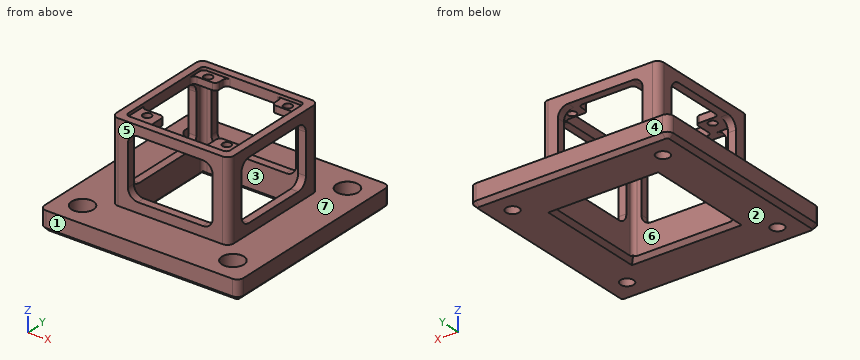
from build123d import *

# Parameters (mm, degrees)
SKETCH2_W                                    = 100
SKETCH2_H                                    = 100
SKETCH2_W_2                                  = 51.2
SKETCH2_H_2                                  = 51.2
BOSS_EXTRUDE1_DEPTH                          = 10
CBORE_FOR_M6_HEX_SOCKET_HEAD_CAP_SCR_2_COUNT = 2
CBORE_FOR_M6_HEX_SOCKET_HEAD_CAP_SCR_2_PITCH = 75.6
CBORE_FOR_M6_HEX_SOCKET_HEAD_CAP_SCR_3_COUNT = 2
CBORE_FOR_M6_HEX_SOCKET_HEAD_CAP_SCR_3_PITCH = 106.914545315
CBORE_FOR_M6_HEX_SOCKET_HEAD_CAP_SCR_4_COUNT = 2
CBORE_FOR_M6_HEX_SOCKET_HEAD_CAP_SCR_4_PITCH = 75.6
SKETCH7_W                                    = 59
SKETCH7_H                                    = 59
SKETCH7_W_2                                  = 51.2
SKETCH7_H_2                                  = 51.2
BOSS_EXTRUDE2_DEPTH                          = 40
SKETCH8_W                                    = 11.608814293
SKETCH8_H                                    = 6.4
SKETCH8_R                                    = 2.1
BOSS_EXTRUDE3_DEPTH                          = 5
FILLET1_R                                    = 3.2
SKETCH11_W                                   = 42.6
SKETCH11_H                                   = 30
CUT_EXTRUDE2_DEPTH                           = 107.396663482
SKETCH12_W                                   = 42.6
SKETCH12_H                                   = 30
CUT_EXTRUDE3_DEPTH                           = 107.396663482
FILLET3_R                                    = 5
FILLET4_R                                    = 5
CHAMFER2_SIZE                                = 2
CHAMFER3_SIZE                                = 2
SKETCH13_W                                   = 51.2
SKETCH13_H                                   = 51.2
CUT_EXTRUDE4_DEPTH                           = 1.5
FILLET5_R                                    = 2


with BuildPart() as part:
    # Sketch2 → Boss-Extrude1 (new body)
    with BuildSketch(Plane(origin=(0, 0, 0), x_dir=(0, 1, 0), z_dir=(0, 0, 1))):
        Rectangle(SKETCH2_W, SKETCH2_H)
        Rectangle(SKETCH2_W_2, SKETCH2_H_2, mode=Mode.SUBTRACT)
    extrude(amount=BOSS_EXTRUDE1_DEPTH)

    # Sketch6 → CBORE for M6 Hex Socket Head Cap Screw1 (revolve, cut)
    with BuildSketch(Plane(origin=(-37.8, 37.8, 10), x_dir=(0, -1, 0), z_dir=(1, 0, 0))):
        Polygon((0, 0), (0, 10), (3.3, 10), (3.3, 6.4), (5.5, 6.4), (5.5, 0.025), (5.525, 0), align=None)
    cbore_for_m6_hex_socket_head_cap_screw1 = revolve(axis=Axis((-37.8, 37.8, 16.35), (0, 0, -1)), mode=Mode.SUBTRACT)

    # CBORE for M6 Hex Socket Head Cap Scr 2: CBORE for M6 Hex Socket Head Cap Screw1 ×2
    with Locations(*[(i * CBORE_FOR_M6_HEX_SOCKET_HEAD_CAP_SCR_2_PITCH, 0, 0) for i in range(1, CBORE_FOR_M6_HEX_SOCKET_HEAD_CAP_SCR_2_COUNT)]):
        add(cbore_for_m6_hex_socket_head_cap_screw1, mode=Mode.SUBTRACT)

    # CBORE for M6 Hex Socket Head Cap Scr 3: CBORE for M6 Hex Socket Head Cap Screw1 ×2
    with Locations(*[Vector(0.7071067811865475, -0.7071067811865476, 0) * (i * CBORE_FOR_M6_HEX_SOCKET_HEAD_CAP_SCR_3_PITCH) for i in range(1, CBORE_FOR_M6_HEX_SOCKET_HEAD_CAP_SCR_3_COUNT)]):
        add(cbore_for_m6_hex_socket_head_cap_screw1, mode=Mode.SUBTRACT)

    # CBORE for M6 Hex Socket Head Cap Scr 4: CBORE for M6 Hex Socket Head Cap Screw1 ×2
    with Locations(*[(0, -i * CBORE_FOR_M6_HEX_SOCKET_HEAD_CAP_SCR_4_PITCH, 0) for i in range(1, CBORE_FOR_M6_HEX_SOCKET_HEAD_CAP_SCR_4_COUNT)]):
        add(cbore_for_m6_hex_socket_head_cap_screw1, mode=Mode.SUBTRACT)

    # Sketch7 → Boss-Extrude2 (add)
    with BuildSketch(Plane.XY.offset(10)):
        Rectangle(SKETCH7_W, SKETCH7_H)
        Rectangle(SKETCH7_W_2, SKETCH7_H_2, mode=Mode.SUBTRACT)
    extrude(amount=BOSS_EXTRUDE2_DEPTH)

    # Sketch8 → Boss-Extrude3 (add)
    # profile 1 of 4: a face of its own
    with BuildSketch(Plane.XY.offset(50)):
        Polygon((13.991185707, -25.6), (20, -25.6), (25.6, -25.6), (25.6, -17.5), (25.6, -15.6), (13.991185707, -15.6), (13.991185707, -17.5), align=None)
        with BuildLine():
            ThreePointArc((22.1, -18.5), (21.48492424, -19.98492424), (20, -20.6))
            ThreePointArc((20, -20.6), (18.51507576, -17.01507576), (22.1, -18.5))
        make_face(mode=Mode.SUBTRACT)
    # profile 2 of 4: a face of its own
    with BuildSketch(Plane.XY.offset(50)):
        Polygon((-20, -25.6), (-13.991185707, -25.6), (-13.991185707, -17.5), (-13.991185707, -15), (-25.6, -15), (-25.6, -17.5), (-25.6, -25.6), align=None)
        with BuildLine():
            ThreePointArc((-17.9, -18.5), (-18.51507576, -19.98492424), (-20, -20.6))
            ThreePointArc((-20, -20.6), (-21.48492424, -17.01507576), (-17.9, -18.5))
        make_face(mode=Mode.SUBTRACT)
    # profile 3 of 4: a face of its own
    with BuildSketch(Plane.XY.offset(50)):
        Polygon((19.986052448, 25.6), (13.991185707, 25.6), (13.991185707, 19.2), (25.6, 19.2), (25.6, 25.6), align=None)
        with BuildLine():
            ThreePointArc((22.086052448, 21.9), (18.501128208, 20.41507576), (19.986052448, 24))
            ThreePointArc((19.986052448, 24), (21.470976689, 23.38492424), (22.086052448, 21.9))
        make_face(mode=Mode.SUBTRACT)
    # profile 4 of 4: a face of its own
    with BuildSketch(Plane.XY.offset(50)):
        with Locations((-19.795592854, 22.4)):
            Rectangle(SKETCH8_W, SKETCH8_H)
        with Locations((-20.013947552, 21.800522552)):
            Circle(SKETCH8_R, mode=Mode.SUBTRACT)
    extrude(amount=-BOSS_EXTRUDE3_DEPTH)

    # Fillet1
    fillet1_edges = [part.edges().sort_by_distance(p)[0] for p in [
        (-29.5, -29.5, 30),
        (29.5, -29.5, 30),
        (50, -50, 5),
        (29.5, 29.5, 30),
        (-50, -50, 5),
        (-50, 50, 5),
        (-29.5, 29.5, 30),
        (50, 50, 5),
    ]]
    fillet(fillet1_edges, radius=FILLET1_R)

    # Sketch11 → Cut-Extrude2 (cut, through all)
    with BuildSketch(Plane(origin=(-29.5, 0, 0), x_dir=(0, -1, 0), z_dir=(-1, 0, 0))):
        with Locations((0, 30)):
            Rectangle(SKETCH11_W, SKETCH11_H)
    extrude(amount=-CUT_EXTRUDE2_DEPTH, mode=Mode.SUBTRACT)

    # Sketch12 → Cut-Extrude3 (cut, through all)
    with BuildSketch(Plane.XZ.offset(29.5)):
        with Locations((0, 30)):
            Rectangle(SKETCH12_W, SKETCH12_H)
    extrude(amount=-CUT_EXTRUDE3_DEPTH, mode=Mode.SUBTRACT)

    # Fillet3
    # the kernel refuses this fillet: 5 mm, written as the material it adds along each edge
    with BuildSketch(Plane(origin=(-29.5, -21.3, 15), x_dir=(0, 1, 0), z_dir=(1, 0, 0)), Plane(origin=(-29.5, -21.3, 45), x_dir=(0, 0, -1), z_dir=(1, 0, 0)), Plane(origin=(25.6, -21.3, 45), x_dir=(0, 0, -1), z_dir=(1, 0, 0)), Plane(origin=(-21.3, -29.5, 15), x_dir=(0, 0, 1), z_dir=(0, 1, 0)), Plane(origin=(21.3, 25.6, 45), x_dir=(0, 0, -1), z_dir=(0, 1, 0))) as fillet3_piece_1:
        with BuildLine():
            CenterArc((FILLET3_R, FILLET3_R), FILLET3_R, 180, 90)
            Line((0, FILLET3_R), (0, 0))
            Line((0, 0), (FILLET3_R, 0))
        make_face()
    extrude(amount=3.9)
    with BuildSketch(Plane(origin=(25.6, -21.3, 15), x_dir=(0, 0, 1), z_dir=(1, 0, 0)), Plane(origin=(25.6, 21.3, 15), x_dir=(0, -1, 0), z_dir=(1, 0, 0)), Plane(origin=(25.6, 21.3, 45), x_dir=(0, 0, -1), z_dir=(1, 0, 0)), Plane(origin=(-21.3, -29.5, 45), x_dir=(0, 0, -1), z_dir=(0, 1, 0)), Plane(origin=(-21.3, 25.6, 45), x_dir=(0, 0, -1), z_dir=(0, 1, 0)), Plane(origin=(21.3, 25.6, 15), x_dir=(0, 0, 1), z_dir=(0, 1, 0)), Plane(origin=(-21.3, 25.6, 15), x_dir=(1, 0, 0), z_dir=(0, 1, 0))) as fillet3_piece_2:
        with BuildLine():
            CenterArc((FILLET3_R, -FILLET3_R), FILLET3_R, 90, 90)
            Line((0, -FILLET3_R), (0, 0))
            Line((0, 0), (FILLET3_R, 0))
        make_face()
    extrude(amount=3.9)

    # Fillet4
    # the kernel refuses this fillet: 5 mm, written as the material it adds along each edge
    with BuildSketch(Plane(origin=(-29.5, 21.3, 15), x_dir=(0, 0, 1), z_dir=(1, 0, 0)), Plane(origin=(21.3, -29.5, 45), x_dir=(0, 0, -1), z_dir=(0, 1, 0))) as fillet4_piece_1:
        with BuildLine():
            CenterArc((FILLET4_R, FILLET4_R), FILLET4_R, 180, 90)
            Line((0, FILLET4_R), (0, 0))
            Line((0, 0), (FILLET4_R, 0))
        make_face()
    extrude(amount=3.9)
    with BuildSketch(Plane(origin=(-29.5, 21.3, 45), x_dir=(0, 0, -1), z_dir=(1, 0, 0)), Plane(origin=(21.3, -29.5, 15), x_dir=(0, 0, 1), z_dir=(0, 1, 0))) as fillet4_piece_2:
        with BuildLine():
            CenterArc((FILLET4_R, -FILLET4_R), FILLET4_R, 90, 90)
            Line((0, -FILLET4_R), (0, 0))
            Line((0, 0), (FILLET4_R, 0))
        make_face()
    extrude(amount=3.9)

    # Chamfer2
    chamfer2_edges = [part.edges().sort_by_distance(p)[0] for p in [
        (0, -50, 0),
        (50, 0, 0),
        (-50, 0, 0),
        (0, 50, 0),
        (-49.0627417, 49.0627417, 0),
        (49.0627417, 49.0627417, 0),
        (49.0627417, -49.0627417, 0),
        (-49.0627417, -49.0627417, 0),
    ]]
    chamfer(chamfer2_edges, length=CHAMFER2_SIZE)

    # Chamfer3
    chamfer3_edges = [part.edges().sort_by_distance(p)[0] for p in [
        (25.6, 0, 0),
        (0, 25.6, 0),
        (0, -25.6, 0),
        (-25.6, 0, 0),
    ]]
    chamfer(chamfer3_edges, length=CHAMFER3_SIZE)

    # Sketch13 → Cut-Extrude4 (cut)
    with BuildSketch(Plane.XY.offset(50)):
        Rectangle(SKETCH13_W, SKETCH13_H)
    extrude(amount=-CUT_EXTRUDE4_DEPTH, mode=Mode.SUBTRACT)

    # Fillet5
    fillet5_edges = [part.edges().sort_by_distance(p)[0] for p in [
        (-25.6, -25.6, 23.5),
        (25.6, -25.6, 23.5),
        (-25.6, 25.6, 23.5),
        (25.6, 25.6, 23.5),
        (-25.6, -15, 46.75),
        (-13.991185707, -15, 46.75),
        (-13.991185707, -25.6, 46.75),
        (13.991185707, -25.6, 46.75),
        (13.991185707, -15.6, 46.75),
        (25.6, -15.6, 46.75),
        (25.6, 19.2, 46.75),
        (13.991185707, 19.2, 46.75),
        (13.991185707, 25.6, 46.75),
        (-13.991185707, 19.2, 46.75),
        (-25.6, 19.2, 46.75),
        (-13.991185707, 25.6, 46.75),
        (25.6, 25.6, 49.25),
        (-25.6, -25.6, 49.25),
        (25.6, -25.6, 49.25),
        (-25.6, 25.6, 49.25),
    ]]
    fillet(fillet5_edges, radius=FILLET5_R)


solid = part.part
The model under review builds one solid part; all positions refer to its coordinate system, in mm. Face numbers are marked on the shaded views. A direction names the side the tool comes from. Coordinates: 2 decimals unless noted, no trailing zeros. Order: outer loops, then holes, each group sorted by start corner. A loop starts at its lowest first (then second) coordinate and runs counter-clockwise, first axis right, second up. Notation, with made-up numbers: (-14, 61.5) -> (24, 61.5) arc R16 cw to (24, 92.5) -> close; hole circle Ø5 at (34, 33.25). An arc over 180 degrees is marked (long way). Answer in a Markdown table with one row per item.
(1) Consider section A-A (x = -37.8). Write out the cut boundary in (y, z) (3 decimals), plus the area to 3 significant figures.
Answers:
| item | result |
|---|---|
| outline | (-50, 2) -> (-48, 0) -> (-41.1, 0) -> (-41.1, 3.6) -> (-43.3, 3.6) -> (-43.3, 9.975) -> (-43.325, 10) -> (-50, 10) -> close; (-34.5, 0) -> (34.5, 0) -> (34.5, 3.6) -> (32.3, 3.6) -> (32.3, 9.975) -> (32.275, 10) -> (-32.275, 10) -> (-32.3, 9.975) -> (-32.3, 3.6) -> (-34.5, 3.6) -> close; (41.1, 0) -> (48, 0) -> (50, 2) -> (50, 10) -> (43.325, 10) -> (43.3, 9.975) -> (43.3, 3.6) -> (41.1, 3.6) -> close |
| area | 808 mm² |
(2) Machinability: for the marked faces 4, 5, 6 and 7, which of the approach directions +Z, -Z, +X, -X, +Y, -Y give a long, thin tool a straight path to every point of the face, cutting with its end or side? Answer none if there is none.
Answers:
| item | result |
|---|---|
| face 4 | +Z, -Z, +X, -X, +Y |
| face 5 | +Z, +X, -X, -Y |
| face 6 | -Z |
| face 7 | +Z |
(3) Consider section B-B (z = 38.5). State how many separate pieces and enclosed holes the cut face has, plus the area to 3 significant figures.
Answers:
| item | result |
|---|---|
| separate pieces | 4 |
| enclosed holes | 0 |
| area | 190 mm² |
(4) The part is to be moulded in two halves that separate along Y. For the marked faces 1, 2 and 3, say which applies: +Y half, -Y half, draft (parallel to the pull), parting line (faces both ways), or undercut.
Answers:
| item | result |
|---|---|
| face 1 | -Y half |
| face 2 | draft |
| face 3 | undercut |
(5) Consider section D-D (y = -11.5). Write out the cut boundary in (x, z), plus the area to 3 significant figures.
Answers:
| item | result |
|---|---|
| outline | (-50, 2) -> (-48, 0) -> (-27.6, 0) -> (-25.6, 2) -> (-25.6, 15) -> (-29.5, 15) -> (-29.5, 10) -> (-50, 10) -> close; (-29.5, 45) -> (-25.6, 45) -> (-25.6, 50) -> (-29.5, 50) -> close; (25.6, 2) -> (27.6, 0) -> (48, 0) -> (50, 2) -> (50, 10) -> (29.5, 10) -> (29.5, 15) -> (25.6, 15) -> close; (25.6, 45) -> (29.5, 45) -> (29.5, 50) -> (25.6, 50) -> close |
| area | 558 mm² |
(6) Wall thickness on line 1 along Y through (x, z) = (-20, 45.8); line 2 along Y through (x, z) = (37.8, 7.5); line 3 along Y through (x, z) = (-26, 21): over which ranges is each line inside the solid? List them lowest first.
Answers:
| item | result |
|---|---|
| line 1 | -29.5 to -20.6, -16.4 to -15, 19.2 to 19.7, 23.9 to 29.5 |
| line 2 | -50 to -43.3, -32.3 to 32.3, 43.3 to 50 |
| line 3 | -29.5 to -21.3, 21.3 to 29.5 |
(7) Insertion check: pin 1 (9 mm diameter, centred on x = -38, y = 39, fed in from +Z); pin 2 (23 mm diameter, centred on x = 9, y = -8.5, fed in from -Z); pin 3 (6.5 mm diameter, centred on x = 20, y = -18.5, fed in from +Z). Each pin has a flat end and moves straight along its axis. Give the tip position at first contact, or say it passes through.
Answers:
| item | result |
|---|---|
| pin 1 | z = 10 |
| pin 2 | z = 45 |
| pin 3 | z = 48.5 |
